The drawing under review shows one solid part. Ordinate dimensions are in mm from its lowest x, y, z. A direction names the side the tool comes from. Coordinates: 2 decimals unless noted, no trailing zeros. Write each loop counter-clockwise with the first axis right and the second up, starting at its lowest first coordinate (ties: lowest second). Pieces come first, ordered by that corner, then holes. Notation, with made-up numbers: (5, -12) - (59, -12) arc R17 cw to (59, 10) - close; hole circle Ø3 at (53.25, -34.75). An arc over 180 degrees is marked (long way). Put each result on its own line as item: value. Start each with the question number.
Item 1: Machinability: for the marked faces 4, 5 and 6, which of the approach directions +Z, -Z, +X, -X, +Y, -Y give a long, thin tool a straight path to every point of the face, cutting with its end or side? Answer none if there is none.
Item 2: To check wall thickness, follow L1, parallel to Z at x = 1.8, y = 2.3; L2, parallel to Z at x = 2.75, y = 4.95; L3, parallel to Y at x = 1.1, z = 1.75. State the ranges of each line that lie inside material, in increasing order. Write a range as [from, to].
Item 3: Consider section A-A on y = 3.65. Give the boundary of the cut face in (x, z), then the cut area to 3 significant figures.
Item 4: Consider section C-C on z = 2.5. Give the boundary of the cut face in (x, y).
Item 5: Mouldability with a two-part tool opening along Z and no side actions: class the marked faces 1, 2 and 3 as pulls with the +Z half, pulls with the -Z half, needs draft (parallel to the pull), parting line crosses it, or undercut.
Item 6: Consider section B-B on x = 3. Give the boundary of the cut face in (y, z), then the cut area to 3 significant figures.
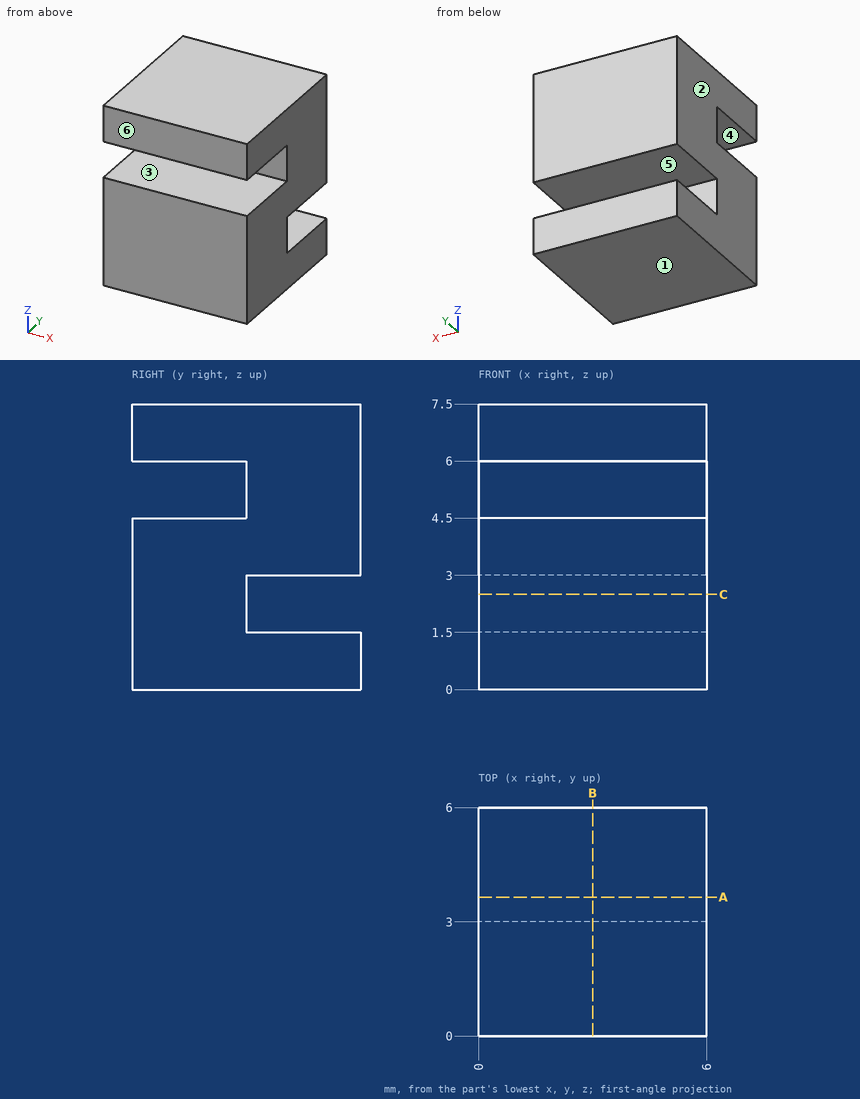
Report:
1. face 4: +X, -X, -Y
1. face 5: +X, -X, +Y
1. face 6: +Z, -Z, +X, -X, -Y
2. L1: [0, 4.5], [6, 7.5]
2. L2: [0, 1.5], [3, 7.5]
2. L3: [0, 3]
3. outline: (0, 0) - (6, 0) - (6, 1.5) - (0, 1.5) - close; (0, 3) - (6, 3) - (6, 7.5) - (0, 7.5) - close
3. area: 36.0 mm²
4. outline: (0, 0) - (6, 0) - (6, 3) - (0, 3) - close
5. face 1: pulls with the -Z half
5. face 2: needs draft
5. face 3: undercut
6. outline: (0, 0) - (6, 0) - (6, 1.5) - (3, 1.5) - (3, 3) - (6, 3) - (6, 7.5) - (0, 7.5) - (0, 6) - (3, 6) - (3, 4.5) - (0, 4.5) - close
6. area: 36.0 mm²
